```python
from build123d import *

# Parameters (mm, degrees)
F0_R     = 3
F1_DEPTH = 5


with BuildPart() as f1:
    # F0 (on Front) → F1 (new body)
    with BuildSketch(Plane.XZ):
        with BuildLine():
            ThreePointArc((12.565296, -30.565649), (14.746833, -30.198005), (16.873467, -30.807674))
            ThreePointArc((16.873467, -30.807674), (25.97897, -29.828457), (28.199125, -20.94364))
            ThreePointArc((28.199125, -20.94364), (27.887223, -18.753438), (28.550916, -16.64304))
            ThreePointArc((28.550916, -16.64304), (31.070939, 11.257989), (11.263325, 31.069005))
            ThreePointArc((11.263325, 31.069005), (8.977661, 32.756053), (7.979957, 35.415936))
            ThreePointArc((7.979957, 35.415936), (0, 42.85), (-7.979957, 35.415936))
            ThreePointArc((-7.979957, 35.415936), (-8.977661, 32.756053), (-11.263325, 31.069005))
            ThreePointArc((-11.263325, 31.069005), (-24.513088, 22.164252), (-32.042752, 8.087498))
            ThreePointArc((-32.042752, 8.087498), (-33.491826, 5.644022), (-36.038116, 4.38434))
            ThreePointArc((-36.038116, 4.38434), (-42.633541, -4.301591), (-34.435945, -11.494952))
            ThreePointArc((-34.435945, -11.494952), (-31.689342, -12.220598), (-29.781365, -14.325358))
            ThreePointArc((-29.781365, -14.325358), (-11.833639, -30.856289), (12.565296, -30.565649))
        make_face()
        with Locations((-34.673953, -3.498494)):
            Circle(F0_R, mode=Mode.SUBTRACT)
        with Locations((20.7248, -23.795739)):
            Circle(F0_R, mode=Mode.SUBTRACT)
        with Locations((0, 34.85)):
            Circle(F0_R, mode=Mode.SUBTRACT)
    extrude(amount=F1_DEPTH)


solid = f1.part
```
Can you work these out from the model? Positions are in its coordinate system, mm. Give positions to 0.01 mm unless a question says otherwise; leave off trailing zeros. Write each loop counter-clockwise with the first axis right and the second up, starting at its lowest first coordinate (ties: lowest second). Pieces come first, ordered by that corner, then holes. Notation, with made-up numbers: (8, 19.5) -> (65, 19.5) arc R17 ccw to (65, 44.5) -> close; hole circle Ø11 at (84.25, 69.5). An arc over 180 degrees is marked (long way). One line per item, written item: value.
Q1. For P1, Ø3, axis at x = -21.5, y = -2, coming from the -Z side; P2, Ø3, axis at y = -2.5, z = 12.5, coming from the -X side, each with a flat end and sliding along its axis, tell me the tip position at first contact or that it passes through.
Results found:
P1: stops at z = -26.31
P2: stops at x = -31.16
Q2. We'd pull the mould along X, two halves only. Please class faces 1 (the face through (0.17, -2.46, 42.85)), 2 (the face through (3, -5, 5)), 3 (the face through (-37.67, -2.46, -3.37)): +X half, -X half, draft (parallel to the pull), parting line (faces both ways), or undercut.
Results found:
face 1: parting line
face 2: draft
face 3: undercut
Q3. Imagine slicing it at B-B on y = -3.55. Please give me the cut outline in (x, z).
Results found:
outline: (-36.04, 4.38) arc R8 ccw to (-34.44, -11.49) arc R5 cw to (-29.78, -14.33) arc R33.05 ccw to (12.57, -30.57) arc R5 cw to (16.87, -30.81) arc R8 ccw to (28.2, -20.94) arc R5 cw to (28.55, -16.64) arc R33.05 ccw to (11.26, 31.07) arc R5 cw to (7.98, 35.42) arc R8 ccw to (-7.98, 35.42) arc R5 cw to (-11.26, 31.07) arc R33.05 ccw to (-32.04, 8.09) arc R5 cw to start; hole circle Ø6 at (-34.67, -3.5); hole circle Ø6 at (0, 34.85); hole circle Ø6 at (20.72, -23.8)
Q4. Imagine slicing it at C-C on z = 21. Please give me the cut outline in (x, y), and give its area (3 significant figures).
Results found:
outline: (-25.52, -5) -> (25.52, -5) -> (25.52, 0) -> (-25.52, 0) -> close
area: 255 mm^2
Q5. Please list where these lines run through material, in increasing order: line 1 (Z direction, x = -2, y = -1.8); line 2 (X direction, y = -4.35, z = -5.5); line 3 (X direction, y = -2.2, z = -3). Write a range as [from, to].
Results found:
line 1: z = [-32.99, 32.61], [37.09, 42.6]
line 2: x = [-42.42, -36.91], [-32.44, 32.59]
line 3: x = [-42.66, -37.63], [-31.72, 32.91]
Q6. Imagine slicing it at D-D on x = -23. Please give me the cut outline in (y, z).
Results found:
outline: (-5, -23.73) -> (0, -23.73) -> (0, 23.73) -> (-5, 23.73) -> close
Q7. Imagine slicing it at A-A on x = 0. Please give me the cut outline in (y, z), and give its area (3 significant figures).
Results found:
outline: (-5, -33.05) -> (0, -33.05) -> (0, 31.85) -> (-5, 31.85) -> close; (-5, 37.85) -> (0, 37.85) -> (0, 42.85) -> (-5, 42.85) -> close
area: 349 mm^2
